Check sheet for the modelled part. Datum: model origin and axes. Units: mm. Face numbers are marked on the shaded views. Round coordinates to 2 decimals unless told otherwise and drop trailing zeros. Write each loop counter-clockwise with the first axis right and the second up, starting at its lowest first coordinate (ties: lowest second). Pieces come first, ordered by that corner, then holes.
Item 1: Section check B-B, the plane y = -37. Record the cut outline in (x, z), plus the area to 3 significant figures.
Item 2: Release check for a two-part mould opening along X. For the marked faces 1, 2 and 3 record: pulls with the +X half, pulls with the -X half, needs draft (parallel to the pull), parting line crosses it, or undercut.
Item 3: Section check C-C, the plane z = 64.5. Record the cut outline in (x, y), plus the area to 3 significant figures.
Item 4: Depth check by flat-ended pin: pin 1 (10 mm diameter, centred on y = -6.5, z = 311.5, fed in from +X); pin 2 (3 mm diameter, centred on y = -36, z = 283, fed in from +X); pin 3 (5 mm diameter, centred on y = -45, z = 329.5, fed in from -X). Enter the tip coordinate at first touch or a pass-through.
Item 5: Section check A-A, the plane z = 292.5. Record the cut outline in (x, y).
Item 6: Material ranges on line 1 along X through (y, z) = (-48, 273); line 2 along Y through (x, z) = (84, 173); line 3 along X through (y, z) = (-40, 208.5), recorded low to high.
Item 7: Section check D-D, the plane x = 226.5. Record the cut outline in (y, z).
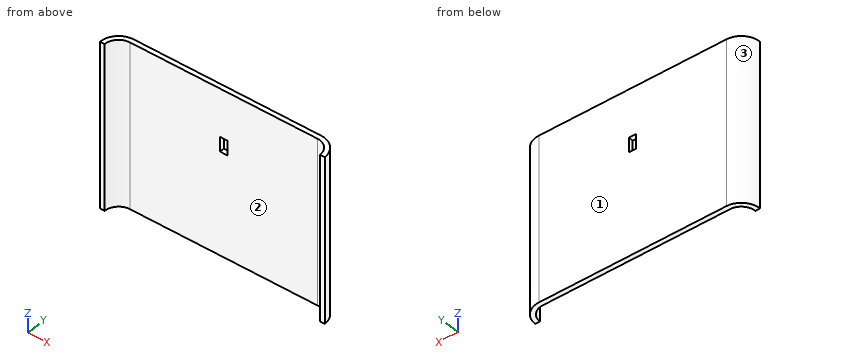
from build123d import *

# Parameters (mm, degrees)
EXTRUDE_THIN1_DEPTH = 457.2
SKETCH5_W           = 19.812
SKETCH5_H           = 40.386
CUT_EXTRUDE1_DEPTH  = 51.8


with BuildPart() as part:
    # Sketch1 → Extrude-Thin1 (new body)
    with BuildSketch(Plane.XY):
        with BuildLine():
            Line((0, 0), (254, 0))
            ThreePointArc((254, 0), (289.921024484, -14.878975516), (304.8, -50.8))
            Line((304.8, -50.8), (292.1, -50.8))
            ThreePointArc((292.1, -50.8), (280.940768363, -23.859231637), (254, -12.7))
            Line((254, -12.7), (0, -12.7))
            Line((0, -12.7), (0, 0))
        make_face()
    extrude_thin1 = extrude(amount=EXTRUDE_THIN1_DEPTH)

    # Mirror1: Extrude-Thin1 across plane
    add(extrude_thin1.mirror(Plane(origin=(0, -12.7, 457.2), x_dir=(0, 0, 1), z_dir=(-1, 0, 0))))

    # Sketch5 → Cut-Extrude1 (cut, through all)
    with BuildSketch(Plane(origin=(0, 0, 0), x_dir=(1, 0, 0), z_dir=(0, 1, 0))):
        with Locations((0, -304.8)):
            Rectangle(SKETCH5_W, SKETCH5_H)
    extrude(amount=-CUT_EXTRUDE1_DEPTH, mode=Mode.SUBTRACT)


solid = part.part
Values found:
1. outline: (-302.89, 0) - (-289.51, 0) - (-289.51, 457.2) - (-302.89, 457.2) - close; (289.51, 0) - (302.89, 0) - (302.89, 457.2) - (289.51, 457.2) - close
1. area: 12,200 mm2
2. face 1: needs draft
2. face 2: undercut
2. face 3: pulls with the -X half
3. outline: (-304.8, -50.8) - (-292.1, -50.8) arc R38.1 cw to (-254, -12.7) - (254, -12.7) arc R38.1 cw to (292.1, -50.8) - (304.8, -50.8) arc R50.8 ccw to (254, 0) - (-254, 0) arc R50.8 ccw to start
3. area: 8,230 mm2
4. pin 1: stops at x = 286.19
4. pin 2: stops at x = 303.03
4. pin 3: stops at x = -304.69
5. outline: (-304.8, -50.8) - (-292.1, -50.8) arc R38.1 cw to (-254, -12.7) - (-9.91, -12.7) - (-9.91, 0) - (-254, 0) arc R50.8 ccw to start; (9.91, -12.7) - (254, -12.7) arc R38.1 cw to (292.1, -50.8) - (304.8, -50.8) arc R50.8 ccw to (254, 0) - (9.91, 0) - close
6. line 1: x = -304.72 to -292, 292 to 304.72
6. line 2: y = -12.7 to 0
6. line 3: x = -303.64 to -290.54, 290.54 to 303.64
7. outline: (-12.7, 0) - (0, 0) - (0, 457.2) - (-12.7, 457.2) - close
